Build history of the part. All positions in model axes, mm. A direction names the side the tool comes from. Give positions to 0.01 mm unless a question says otherwise; leave off trailing zeros. Write each loop counter-clockwise with the first axis right and the second up, starting at its lowest first coordinate (ties: lowest second). Pieces come first, ordered by that corner, then holes. Notation, with made-up numbers: (-20, -24.5) -> (-12, -24.5) arc R15 ccw to (-12, -12.5) -> close; hole circle Ø2 at (-12.5, 21.5). An arc over 180 degrees is marked (long way). Put each result on its own line as item: value.
Autodesk Inventor part; units mm, degrees
ref_plane "YZ Plane" through (0, 0, 0) normal (1, 0, 0) x (0, 1, 0)
ref_plane "XZ Plane" through (0, 0, 0) normal (0, 1, 0) x (-1, 0, 0)
ref_plane "XY Plane" through (0, 0, 0) normal (0, 0, 1) x (1, 0, 0)
sketch "Sketch3" plane through (0, 0, 0) normal (0, 0, 1) x (1, 0, 0)
  line L0 (26, 0) -> (26, 25)
  line L1 (26, 25) -> (2.3151, 25)
  circle A0 centre (2.2, 2.2) radius 2.2
  circle A1 centre (2.2, 2.2) radius 1.1
  circle A2 centre (2.2, 14.7) radius 1.1
  circle A3 centre (2.2, 14.7) radius 2.2
  circle A4 centre (23.2, 2.2) radius 2.2
  circle A5 centre (23.2, 2.2) radius 1.1
  circle A6 centre (23.2, 14.7) radius 1.1
  circle A7 centre (23.2, 14.7) radius 2.2
  line L2 (2.2, 2.2) -> (-0.6, 2.2)
  line L3 (-0.6, 2.2) -> (-0.6, 0)
  line L4 (-0.6, 0) -> (2.2, 0)
  line L5 (2.2, 0) -> (2.2, 2.2)
  line L6 (-0.6, 0) -> (26, 0)
  line L7 (26, 0) -> (26, 25)
  line L8 (26, 25) -> (-0.6, 25)
  line L9 (-0.6, 25) -> (-0.6, 0)
  line L10 (-0.6, 25) -> (26, 25)
  line L11 (26, 25) -> (26, 18)
  line L12 (26, 18) -> (-0.6, 18)
  line L13 (-0.6, 18) -> (-0.6, 25)
  point P0 (0, 0)
  point P1 (-0.6, 18)
  dimension "d14" = 25
  dimension "d15" = 4.4
  dimension "d16" = 2.2
  dimension "d18" = 2.2
  dimension "d19" = 4.4
  dimension "d21" = 4.4
  dimension "d22" = 2.2
  dimension "d23" = 4.4
  dimension "d25" = 7
extrude "Extrusion1" add sketch "Sketch3" along normal blind 3 contours A4 | L6 A0 L2 L9 L12 L0 | L5 A1 L2 A0 | L4 L3 L2 A0 | A0 L2 A1 L5 | A3 | A7
sketch "Sketch5" plane through (0, 0, 3) normal (0, 0, 1) x (1, 0, 0)
  line L0 (26, 0) -> (26, 25)
  line L1 (26, 25) -> (2.3151, 25)
  circle A0 centre (2.2, 2.2) radius 2.2
  circle A1 centre (2.2, 2.2) radius 1.1
  circle A2 centre (2.2, 14.7) radius 1.1
  circle A3 centre (2.2, 14.7) radius 2.2
  circle A4 centre (23.2, 2.2) radius 2.2
  circle A5 centre (23.2, 2.2) radius 1.1
  circle A6 centre (23.2, 14.7) radius 1.1
  circle A7 centre (23.2, 14.7) radius 2.2
  line L2 (2.2, 2.2) -> (-0.6, 2.2)
  line L3 (-0.6, 2.2) -> (-0.6, 0)
  line L4 (-0.6, 0) -> (2.2, 0)
  line L5 (2.2, 0) -> (2.2, 2.2)
  line L6 (-0.6, 0) -> (26, 0)
  line L7 (26, 0) -> (26, 25)
  line L8 (26, 25) -> (-0.6, 25)
  line L9 (-0.6, 25) -> (-0.6, 0)
  line L10 (-0.6, 25) -> (26, 25)
  line L11 (26, 25) -> (26, 18)
  line L12 (26, 18) -> (-0.6, 18)
  line L13 (-0.6, 18) -> (-0.6, 25)
  point P0 (0, 0)
  point P1 (0, 0)
  point P2 (-0.6, 18)
  point P3 (-0.6, 18)
  dimension "d28" = 25
  dimension "d29" = 4.4
  dimension "d30" = 2.2
  dimension "d31" = 2.2
  dimension "d32" = 4.4
  dimension "d33" = 4.4
  dimension "d34" = 2.2
  dimension "d35" = 4.4
  dimension "d36" = 7
extrude "Extrusion2" add sketch "Sketch5" against normal blind 1 contours L12 L9 L8 L1 L0
sketch "Sketch6" plane through (0, 0, 3) normal (0, 0, 1) x (1, 0, 0)
  line L0 (26, 0) -> (26, 25)
  line L1 (26, 25) -> (2.3151, 25)
  circle A0 centre (2.2, 2.2) radius 2.2
  circle A1 centre (2.2, 2.2) radius 1.1
  circle A2 centre (2.2, 14.7) radius 1.1
  circle A3 centre (2.2, 14.7) radius 2.2
  circle A4 centre (23.2, 2.2) radius 2.2
  circle A5 centre (23.2, 2.2) radius 1.1
  circle A6 centre (23.2, 14.7) radius 1.1
  circle A7 centre (23.2, 14.7) radius 2.2
  line L2 (2.2, 2.2) -> (-0.6, 2.2)
  line L3 (-0.6, 2.2) -> (-0.6, 0)
  line L4 (-0.6, 0) -> (2.2, 0)
  line L5 (2.2, 0) -> (2.2, 2.2)
  line L6 (-0.6, 0) -> (26, 0)
  line L7 (26, 0) -> (26, 25)
  line L8 (26, 25) -> (-0.6, 25)
  line L9 (-0.6, 25) -> (-0.6, 0)
  line L10 (-0.6, 25) -> (26, 25)
  line L11 (26, 25) -> (26, 18)
  line L12 (26, 18) -> (-0.6, 18)
  line L13 (-0.6, 18) -> (-0.6, 25)
  point P0 (0, 0)
  point P1 (0, 0)
  point P2 (-0.6, 18)
  dimension "d39" = 25
  dimension "d40" = 4.4
  dimension "d41" = 2.2
  dimension "d42" = 2.2
  dimension "d43" = 4.4
  dimension "d44" = 4.4
  dimension "d45" = 2.2
  dimension "d46" = 4.4
  dimension "d47" = 7
extrude "Extrusion3" add sketch "Sketch6" against normal blind 4.5 contours A4 | L5 A1 L2 A0 | A0 L2 A1 L5 | A3 | A7
fillet "Fillet1" radius 2 6 edges at (26, 25, 2.5) (-0.6, 25, 2.5) (26, 18, 1) (-0.6, 18, 1) (-0.6, 0, 1.5) (26, 0, 1.5)
thread "Thread1"
thread "Thread2"
thread "Thread3"
thread "Thread4"
sketch "Sketch7" plane through (0, 0, 3) normal (0, 0, 1) x (1, 0, 0)
  circle A0 centre (2.2, 2.2) radius 1.1
  circle A1 centre (23.2, 14.7) radius 1.1
  circle A2 centre (2.2, 2.2) radius 2.2
  circle A3 centre (23.2, 14.7) radius 2.2
  line L0 (-0.6, 3.85) -> (26, 3.85)
  line L1 (26, 3.85) -> (26, 13.05)
  line L2 (26, 13.05) -> (-0.6, 13.05)
  line L3 (-0.6, 13.05) -> (-0.6, 3.85)
  point P0 (0, 0)
  point P1 (23.2, 13.05)
  point P2 (2.2, 3.85)
extrude "Extrusion4" cut sketch "Sketch7" against normal blind 1 contours L0 A2 | A2 L0 L3 L2 A3 L1 | A3 L2 picked at (2.5398, 3.9498) picked at (23.5398, 12.9502)
sketch "Sketch8" plane through (0, 0, 2) normal (0, 0, 1) x (1, 0, 0)
  line L0 (-0.6, 3.85) -> (-0.6, 13.05)
  line L1 (-0.6, 13.05) -> (26, 13.05)
  line L2 (-0.6, 3.85) -> (26, 3.85)
  line L3 (26, 3.85) -> (26, 13.05)
  line L4 (26, 13.05) -> (-0.6, 13.05)
  line L5 (-0.6, 13.05) -> (-0.6, 3.85)
  line L6 (26, 3.85) -> (-0.6, 3.85)
  line L7 (12.7, 3.85) -> (14.9828, 3.85)
  line L8 (14.9828, 3.85) -> (12.7, 3.85)
  line L9 (15.7821, 13.05) -> (15.7821, 3.85)
  line L10 (9.7, 3.85) -> (9.7, 13.05)
  point P0 (0, 0)
  point P1 (15.7821, 3.85)
extrude "Extrusion5" add sketch "Sketch8" along normal blind 10 contours L10 L1 L9 L2
fillet "Fillet2" radius 0.3 4 edges at (4.55, 13.05, 3) (4.55, 3.85, 3) (20.8911, 13.05, 3) (20.8911, 3.85, 3)
sketch "Sketch9" plane through (15.7821, 3.85, 2) normal (1, 0, 0) x (0, 0, -1)
  line L0 (0, 0) -> (0, 4.6)
  line L1 (-10, 0) -> (-10, 9.2)
  circle A0 centre (-5, 4.6) radius 1.6
  circle A1 centre (-5, 4.6) radius 2.75
  line L2 (-1, 0) -> (-5, 1.85)
  line L3 (-1, 9.2) -> (-10, 9.2)
  line L4 (-1, 9.2) -> (-5, 7.35)
  line L5 (0, 0) -> (-0.7, 0)
  line L6 (-10, 0) -> (0, 0)
  line L7 (0, 0) -> (0, 9.2)
  line L8 (0, 9.2) -> (-1, 9.2)
  line L9 (-0.7, 9.2) -> (0, 9.2)
  line L10 (-1, 0) -> (-1, -0.3)
  arc A2 (-1, 0) -> (-5, 1.85) centre (-4.8841, -3.1487) ccw
  arc A3 (-5, 7.35) -> (-1, 9.2) centre (-4.8841, 12.3487) ccw
  point P0 (2, -3.85)
  point P1 (-4.9177, 7.3488)
  point P2 (-4.9177, 1.8512)
  dimension "d69" = 3.2
  dimension "d70" = 5.5
  dimension "d73" = 5
  dimension "d74" = 5
extrude "Extrusion6" cut sketch "Sketch9" against normal blind 10 contours L6 L1 L3 L4 A1 L2 | L2 A2 | A3 L4
sketch "Sketch10" plane through (15.7821, 3.85, 2) normal (1, 0, 0) x (0, 0, -1)
  line L0 (0, 0) -> (0, 4.6)
  line L1 (-10, 0) -> (-10, 9.2)
  circle A0 centre (-5, 4.6) radius 1.6
  circle A1 centre (-5, 4.6) radius 2.75
  line L2 (-1, 0) -> (-5, 1.85)
  line L3 (-1, 9.2) -> (-10, 9.2)
  line L4 (-1, 9.2) -> (-5, 7.35)
  line L5 (0, 0) -> (-0.7, 0)
  line L6 (-10, 0) -> (0, 0)
  line L7 (0, 0) -> (0, 9.2)
  line L8 (0, 9.2) -> (-1, 9.2)
  line L9 (-0.7, 9.2) -> (0, 9.2)
  line L10 (-1, 0) -> (-1, -0.3)
  arc A2 (-1, 0) -> (-5, 1.85) centre (-4.8841, -3.1487) ccw
  arc A3 (-5, 7.35) -> (-1, 9.2) centre (-4.8841, 12.3487) ccw
  point P0 (2, -3.85)
  point P1 (2, -3.85)
  point P2 (-4.9177, 7.3488)
  point P3 (-4.9177, 1.8512)
  dimension "d75" = 3.2
  dimension "d76" = 5.5
  dimension "d77" = 5
  dimension "d78" = 5
extrude "Extrusion7" cut sketch "Sketch10" against normal blind 10 contours A0
thread "Thread5"
properties part number "supCamnovo"
1) Pin check, flat tips, straight feed: pin 1 (2 mm diameter, centred on x = 2.2, y = 2.2, fed in from +Z); pin 2 (4.5 mm diameter, centred on x = 21.5, y = 6.5, fed in from +Z); pin 3 (0.6 mm diameter, centred on x = 20.5, z = 2.5, fed in from -Y); pin 4 (1 mm diameter, centred on y = 5, z = 5, fed in from -X). Stop position of each tip, or through.
Filled sheet:
pin 1: through
pin 2: z = 2
pin 3: y = 0
pin 4: x = 9.7
2) Slice it at D-D (z = 6.5). Write the cut outline in (x, y), plus the area to 3 significant figures.
Filled sheet:
outline: (9.7, 5.69) -> (15.78, 5.69) -> (15.78, 6.93) -> (9.7, 6.93) -> close; (9.7, 9.97) -> (15.78, 9.97) -> (15.78, 11.21) -> (9.7, 11.21) -> close
area: 15.1 mm2
3) Tool access for faces 4 (the flat face through (13, 19, 3)), 5 (the flat face through (13, 18, 1)), 6 (the cylindrical face through (21.454, 13.361, -0.74)): list every direction of +Z, -Z, +X, -X, +Y, -Y with a clear straight run to the whole face (end or side of a thin tool).
Filled sheet:
face 4: +Z, +X, -X, +Y
face 5: -Z, +X, -X, +Y
face 6: -Z
4) Pull direction Y, two halves, no side cores. Call faces 1 (the flat face through (3, 16, -1.5)), 2 (the cylindrical face through (2.06, 13.61, 0.72)), 3 (the cylindrical face through (0, 17.43, 1.01)): released by +Y, released by -Y, zero draft, split by the parting line, or undercut.
Filled sheet:
face 1: zero draft
face 2: undercut
face 3: released by +Y
5) Slice it at A-A (y = 8.45). Write the cut outline in (x, z), plus the area to 3 significant figures.
Filled sheet:
outline: (-0.6, 0) -> (26, 0) -> (26, 2) -> (15.78, 2) -> (15.78, 5.4) -> (9.7, 5.4) -> (9.7, 2) -> (-0.6, 2) -> close; (9.7, 8.6) -> (15.78, 8.6) -> (15.78, 9.75) -> (9.7, 9.75) -> close
area: 80.9 mm2
6) Slice it at C-C (y = 14.7). Write the cut outline in (x, z).
Filled sheet:
outline: (-0.6, 0) -> (0, 0) -> (0, -1.5) -> (1.1, -1.5) -> (1.1, 3) -> (-0.6, 3) -> close; (3.3, -1.5) -> (4.4, -1.5) -> (4.4, 0) -> (21, 0) -> (21, -1.5) -> (22.1, -1.5) -> (22.1, 3) -> (3.3, 3) -> close; (24.3, -1.5) -> (25.4, -1.5) -> (25.4, 0) -> (26, 0) -> (26, 3) -> (24.3, 3) -> close
7) Slice it at B-B (x = 10.75). Write the cut outline in (y, z).
Filled sheet:
outline: (0, 0) -> (18, 0) -> (18, 2) -> (25, 2) -> (25, 3) -> (13.05, 3) arc R5 cw to (11.2, 7) arc R2.75 ccw to (5.7, 7) arc R5 cw to (3.85, 3) -> (0, 3) -> close; hole circle Ø3.2 at (8.45, 7)
8) Wall check: L1, parallel to Y at x = 23.2, z = 0.05; L2, parallel to Y at x = 9.25, z = 2.25; L3, parallel to Z at x = 5.25, y = 21.5. Give the ranges that are in metal, low to high.
Filled sheet:
L1: 0 to 1.1, 3.3 to 13.6, 15.8 to 18
L2: 0 to 3.85, 13.05 to 25
L3: 2 to 3
